The listing builds one solid part. Answer for the finished solid, in the listing's coordinates (mm). A direction names the side the tool comes from. Give positions to 0.01 mm unless a question says otherwise; leave off trailing zeros. Order: outer loops, then holes, each group sorted by start corner. A loop starts at its lowest first (then second) coordinate and runs counter-clockwise, first axis right, second up. Notation, with made-up numbers: (41.5, -7.75) - (74.5, -7.75) arc R12 cw to (74.5, -2.75) - close; hole circle Ø7 at (-40, -25.75). An arc over 180 degrees is marked (long way). Write each question's results on one line, items separated by ' | '. Start each with the question number.
1. Determine the mould class of faces 1 (the face through (-49, 4, -5)), 2 (the face through (24.336, -0.715, -16.246)), 3 (the face through (-56.605, 4.295, -4.19)), 4 (the face through (12.14, -0.24, 1.66)) for opening direction X: released by +X, released by -X, zero draft, split by the parting line, or undercut.
2. Which of the six approach directions +Z, -Z, +X, -X, +Y, -Y give full straight-line access (tool end or side, diameter ignored) to faces 5 (the face through (-56.605, -4.19, -4.295)), 6 (the face through (-56.605, -4.295, 4.19)), 7 (the face through (-56.605, 4.19, 4.295)), 8 (the face through (-64, 0, 0)), 9 (the face through (0, 8, -8))?
3. Flat-ended cylindrical pins translate along their axes: pin 1 (5 mm diameter, centred on x = 2.5, z = 2, fed in from +Y); pin 2 (1.5 mm diameter, centred on x = 30, y = 10, fed in from +Z); pin 3 (1 mm diameter, centred on y = -7.5, z = 12.5, fed in from -X). Find the tip coordinate at first contact, or state that the pin passes through.
4. Section B-B (x = -25) is taken. Give the vertices of the cut face in (y, z), and give its area (3 significant figures).
5. Find the intervals of material crossed by L1, parallel to X at y = 4, z = 0; L2, parallel to X at y = 9, z = 0; L3, parallel to Y at x = -18.5, z = 0.5, in increasing order.
6. Section C-C (x = 9.5) is taken. Give the vertices of the cut face in (y, z), and give its area (3 significant figures).
7. Section A-A (x = 22) is taken. Give the vertices of the cut face in (y, z).
from build123d import *

# Parameters (mm, degrees)
CUT_EXTRUDE_1_DEPTH      = 69.876701431
CUT_EXTRUDE_1_DEPTH_BACK = 69.876701431
SKETCH_2_R               = 10
SKETCH_3_OUTSIDE_W       = 62.606
SKETCH_3_OUTSIDE_H       = 62.606
CUT_EXTRUDE_2_DEPTH      = 15
CHAMFER_1_SIZE           = 1


with BuildPart() as part:
    # 草图1 → 旋转1 (revolve)
    with BuildSketch(Plane.XY, mode=Mode.PRIVATE) as revolve_1_sk:
        Polygon((-64, 0), (-64, 8), (-49, 8), (-49, 10), (0, 10), (0, 18), (48, 14.571428571), (48, 0), align=None)
    revolve(revolve_1_sk.sketch.rotate(Axis((-69.993580533, 0, 0), (1, 0, 0)), 90), axis=Axis((-69.993580533, 0, 0), (1, 0, 0)))

    # 草图2 → 拉伸1 (cut, two sides: drawn at the far end of the back side and taken through both)
    with BuildSketch(Plane(origin=(0, 0, 0), x_dir=(1, 0, 0), z_dir=(0, 1, 0)).offset(-CUT_EXTRUDE_1_DEPTH_BACK)):
        with Locations(Location((22, 0, 0), (0, 0, 132.082422816))):
            Circle(SKETCH_2_R)
    extrude(amount=CUT_EXTRUDE_1_DEPTH + CUT_EXTRUDE_1_DEPTH_BACK, mode=Mode.SUBTRACT)

    # 草图3 outside → 拉伸2 (cut)
    with BuildSketch(Plane.ZY.offset(64)):
        Rectangle(SKETCH_3_OUTSIDE_W, SKETCH_3_OUTSIDE_H)
        Polygon((-8.485281374, 0), (0, -8.485281374), (8.485281374, 0), (0, 8.485281374), align=None, mode=Mode.SUBTRACT)
    extrude(amount=-CUT_EXTRUDE_2_DEPTH, mode=Mode.SUBTRACT)

    # 倒角1
    chamfer_1_edges = [part.edges().sort_by_distance(p)[0] for p in [
        (-49, 0, -10),
    ]]
    chamfer(chamfer_1_edges, length=CHAMFER_1_SIZE)


solid = part.part
Reported:
1) face 1: released by -X | face 2: released by +X | face 3: zero draft | face 4: undercut
2) face 5: -Z, -X, -Y | face 6: +Z, -X, -Y | face 7: +Z, -X, +Y | face 8: +Z, -Z, -X, +Y, -Y | face 9: -X
3) pin 1: y = 17.96 | pin 2: z = 12.88 | pin 3: x = 0
4) outline: circle Ø20 at (0, 0) | area: 314 mm²
5) L1: -64 to 12, 32 to 48 | L2: -49 to 12, 32 to 48 | L3: -9.99 to 9.99
6) outline: circle Ø34.64 at (0, 0) | area: 943 mm²
7) outline: (-13.03, -10) arc R16.43 ccw to (13.03, -10) - close; (-13.03, 10) - (13.03, 10) arc R16.43 ccw to start
